Drawing for the job (mm, zero at the part's lowest x, y, z). Round coordinates to 2 decimals unless told otherwise and drop trailing zeros. Write each loop counter-clockwise with the first axis right and the second up, starting at its lowest first coordinate (ties: lowest second). Pieces come first, ordered by that corner, then holes. Notation, with made-up numbers: (81, -11) - (123, -11) arc R16 cw to (123, -5) - close; hole circle Ø4 at (61.25, -14). An arc over 180 degrees is marked (long way). One line per question, with ' | ' between items.
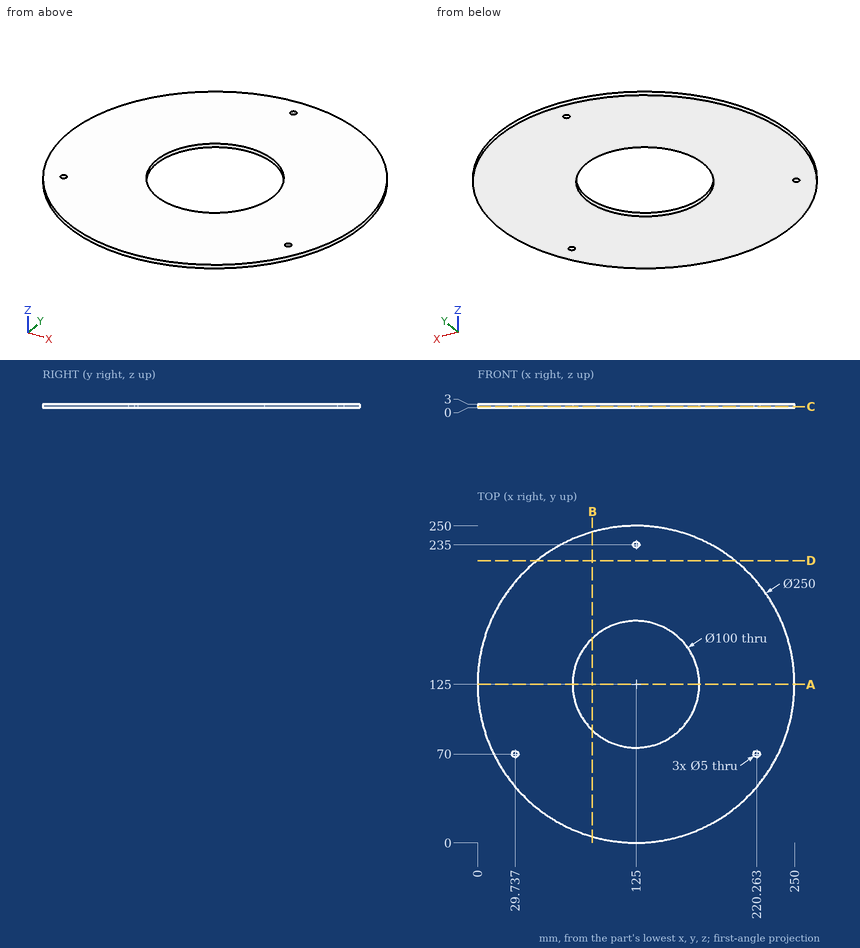
Q1. Saw through at D-D, the plane y = 222.5. List the corners of the cut face in (x, z), then the cut area to 3 significant figures.
Found:
outline: (46.78, 0) - (203.22, 0) - (203.22, 3) - (46.78, 3) - close | area: 469 mm^2
Q2. Saw through at C-C, the plane z = 0.9. List the corners of the cut face in (x, y), then the cut area to 3 significant figures.
Found:
outline: circle Ø250 at (125, 125); hole circle Ø5 at (29.74, 70); hole circle Ø100 at (125, 125); hole circle Ø5 at (125, 235); hole circle Ø5 at (220.26, 70) | area: 41,200 mm^2
Q3. Drill centre lines: L1, parallel to X at y = 99, z = 2.35; L2, parallel to X at y = 139.5, z = 2.55; L3, parallel to Y at x = 39, z = 2.75 (1 decimal). Where is each one in solid material? Low to high. Write a range as from..to.
Found:
L1: 2.73..82.29, 167.71..247.27 | L2: 0.84..77.15, 172.85..249.16 | L3: 34.3..215.7
Q4. Drop flat-ended pins along their axis: pin 1 (3 mm diameter, centred on x = 29.74, y = 70, fed in from -Z); pin 2 (1 mm diameter, centred on y = 81, z = 1.5, fed in from -X); pin 3 (1 mm diameter, centred on y = 130, z = 0.5, fed in from -X). Give the stop position or say it passes through.
Found:
pin 1: through | pin 2: x = 7.81 | pin 3: x = 0.08
Q5. Saw through at B-B, the plane x = 90.5. List the corners of the cut face in (y, z) (1 decimal).
Found:
outline: (4.9, 0) - (88.8, 0) - (88.8, 3) - (4.9, 3) - close; (161.2, 0) - (245.1, 0) - (245.1, 3) - (161.2, 3) - close
Q6. Saw through at A-A, the plane y = 125. List the corners of the cut face in (x, z), then the cut area to 3 significant figures.
Found:
outline: (0, 0) - (75, 0) - (75, 3) - (0, 3) - close; (175, 0) - (250, 0) - (250, 3) - (175, 3) - close | area: 450 mm^2
